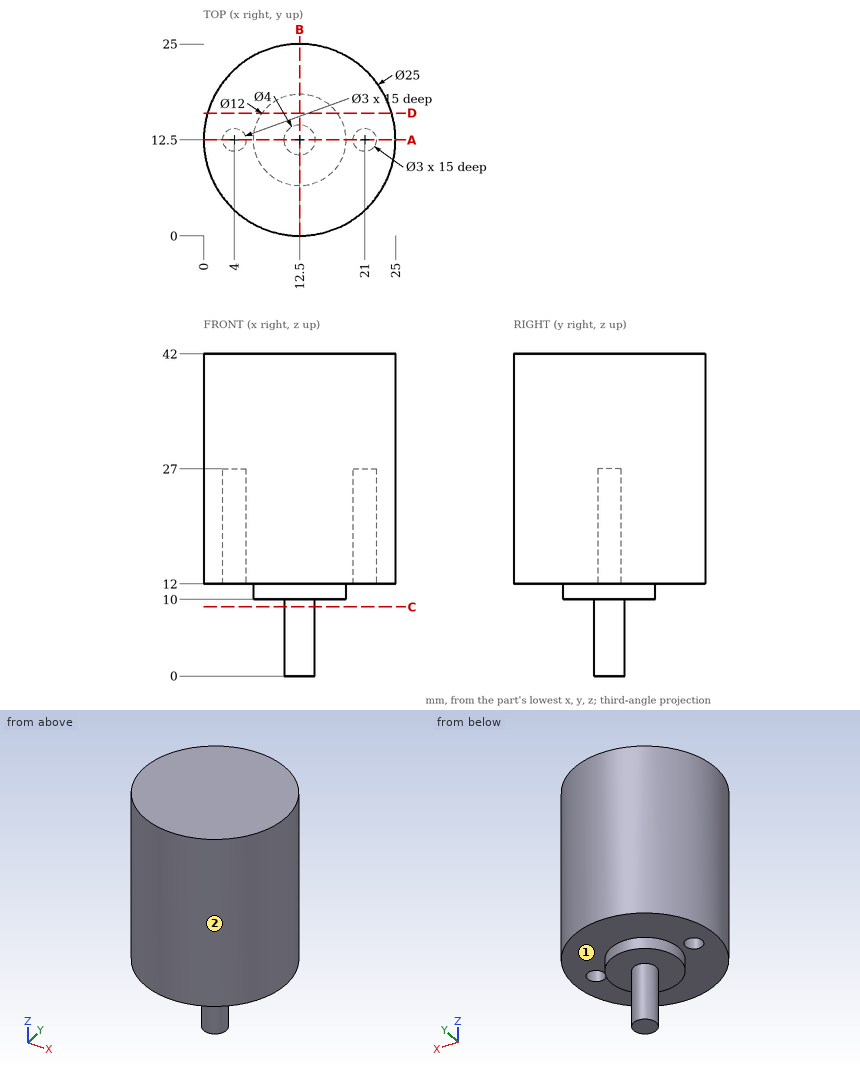
Verification items for this drawing (mm, ordinates from the low corner). A direction names the side the tool comes from. Coordinates: 2 decimals unless noted, no trailing zeros. Loops run counter-clockwise (first coordinate to the right, second up) from the corner with the lowest first, then second, coordinate; pieces in that order, holes last. Notation, with made-up numbers: (-40, 51) - (-34, 51) arc R29 cw to (-34, 72) - close; hole circle Ø9 at (-27.5, -20). An arc over 180 degrees is marked (long way). One line per item, written item: value. Start each with the question number.
(1) Cross-section at A-A on y = 12.5. Enter the section's corners in (x, z).
(2) Material ranges on line 1 (X direction, y = 12.5, z = 11); line 2 (Z direction, x = 6.5, y = 6.25); line 3 (Y direction, x = 21, z = 17.5), recorded low to high. Write a range as [from, to].
(3) Cross-section at C-C on z = 9. Enter the section's corners in (x, y).
(4) Cross-section at D-D on y = 16. Enter the section's corners in (x, z), plus the area to 3 significant figures.
(5) Cross-section at B-B on x = 12.5. Enter the section's corners in (y, z).
(6) Tool access check on the marked faces 1 and 2. Record the directions out of +Z, -Z, +X, -X, +Y, -Y that give a thin tool (end or side, any length) a straight path to the whole face; none if there is none.
(7) Depth check by flat-ended pin: P1, Ø4, axis at x = 14.5, y = 7.5, coming from the -Z side; P2, Ø8, axis at y = 19.5, z = 34, coming from the -X side; P3, Ø4, axis at x = 5, z = 20, coming from the -Y side (3 decimals); P4, Ø6, axis at x = 15.5, y = 10.5, coming from the -Z side. Enter the tip coordinate at first touch or a pass-through.
Results below:
1. outline: (0, 12) - (2.5, 12) - (2.5, 27) - (5.5, 27) - (5.5, 12) - (6.5, 12) - (6.5, 10) - (10.5, 10) - (10.5, 0) - (14.5, 0) - (14.5, 10) - (18.5, 10) - (18.5, 12) - (19.5, 12) - (19.5, 27) - (22.5, 27) - (22.5, 12) - (25, 12) - (25, 42) - (0, 42) - close
2. line 1: x = [6.5, 18.5]
2. line 2: z = [12, 42]
2. line 3: y = [3.33, 11], [14, 21.67]
3. outline: circle Ø4 at (12.5, 12.5)
4. outline: (0.5, 12) - (7.63, 12) - (7.63, 10) - (17.37, 10) - (17.37, 12) - (24.5, 12) - (24.5, 42) - (0.5, 42) - close
4. area: 739 mm2
5. outline: (0, 12) - (6.5, 12) - (6.5, 10) - (10.5, 10) - (10.5, 0) - (14.5, 0) - (14.5, 10) - (18.5, 10) - (18.5, 12) - (25, 12) - (25, 42) - (0, 42) - close
6. face 1: -Z
6. face 2: +Z, -Z
7. P1: stops at z = 10
7. P2: stops at x = 0.37
7. P3: stops at y = 1.275
7. P4: stops at z = 0
